Can you work these out from the model? Positions are in its coordinate system, mm. A direction names the side the tool comes from. Give positions to 0.01 mm unless a question says otherwise; leave off trailing zeros. Loops run counter-clockwise (first coordinate to the right, second up) from the corner with the lowest first, then second, coordinate; pieces in that order, holes last. Notation, with made-up numbers: (71, -8) -> (130, -8) arc R21 cw to (130, 23) -> close; hole circle Ø6 at (73, -25.75). An arc over 180 degrees is marked (long way). Use CSV: the item, a comma, the result in double quotes.
Solid Edge part; units mm, degrees
sketch "Sketch1" plane through (0, 0, 0) normal (1, 0, 0) x (0, 1, 0)
  line L0 (0, 7.4) -> (37.4, 7.4)
  line L1 (37.4, 7.4) -> (37.4, -7.4)
  line L2 (37.4, -7.4) -> (0, -7.4)
  line L3 (0, -7.4) -> (0, 7.4)
  dimension "D1" = 37.4
extrude "Protrusion1" add sketch "Sketch1" along normal mid plane 20
sketch "Sketch2" plane through (0, 0, 0) normal (0, 0, 1) x (1, 0, 0)
  line L0 (-5, 37.4) -> (-5, 46.4)
  line L1 (-5, 46.4) -> (5, 46.4)
  line L2 (5, 37.4) -> (5, 46.4)
extrude "Extrusionsausprägung_2" add sketch "Sketch2" along normal mid plane 7.8 material side at (-4.95, 41.9, 0)
fillet "Verrundung_1" radius 3 2 edges at (5, 46.4, 0) (-5, 46.4, 0)
sketch "Sketch3" plane through (0, 37.4, 0) normal (0, 1, 0) x (0, 0, -1)
  line L0 (-3.9, 5) -> (-3.9, 6.25)
  line L1 (-3.9, 6.25) -> (4.6, 6.25)
  line L2 (4.6, 6.25) -> (4.6, 5)
  line L3 (4.6, 5) -> (-3.9, 5)
  dimension "D1" = 3.9
  dimension "D2" = 3.9
extrude "Extrusionsausprägung_3" add sketch "Sketch3" along normal mid plane 2.39
sketch "Sketch4" plane through (-0.625, 41.9, 3.9) normal (0, 0, 1) x (0, 1, 0)
  circle A0 centre (-0.005, -0.625) radius 2
extrude "Cutout1" cut sketch "Sketch4" along normal mid plane 36
sketch "Sketch5" plane through (0, 18.7, 7.4) normal (0, 0, 1) x (0, 1, 0)
  line L0 (-18.7, 9.1438) -> (-10.3, 9.1438)
  line L1 (-10.3, 9.1438) -> (-8.8895, 10)
  dimension "D1" = 10.3
extrude "Extrusionsausschnitt_2" cut sketch "Sketch5" along normal mid plane 87 material side at (-9.1938, 4.2, 7.4)
sketch "Sketch6" plane through (0.4281, 0, 0) normal (0, -1, 0) x (0, 0, 1)
  circle A0 centre (0, 0.4281) radius 8
extrude "Extrusionsausprägung_4" add sketch "Sketch6" along normal blind 29.1
sketch "Sketch7" plane through (10, 18.7, 0) normal (1, 0, 0) x (0, 1, 0)
  line L0 (-55.4467, 6) -> (-18.7, 6)
  line L1 (-18.7, 6) -> (-18.7, 10.4583)
extrude "Extrusionsausschnitt_3" cut sketch "Sketch7" along normal mid plane 52 material side at (10, -18.3734, 6.05)
mirror "Mirror1" about plane through (0, 0, 0) normal (0, 0, 1) of "Extrusionsausschnitt_3"
sketch "Sketch8" plane through (0, -29.1, 0) normal (0, -1, 0) x (1, 0, 0)
  circle A0 centre (0, 0) radius 4.5
extrude "Extrusionsausschnitt_5" cut sketch "Sketch8" against normal blind 30
(1) If we section it at D-D, the plane x = 7: Write out the boundary of the cut face in (y, z).
Answer sheet:
outline,"(-29.1, -3.87) -> (0, -3.87) -> (0, -7.4) -> (37.4, -7.4) -> (37.4, 7.4) -> (0, 7.4) -> (0, 3.87) -> (-29.1, 3.87) -> close"
(2) If I drill on L1, parallel to Z at x = 0, y = -13; L2, parallel to Y at x = 0, z = 0.75 (3 decimals); L3, parallel to Y at x = 4.25, z = -5, over which ranges is the centre line in solid material (lowest first)? Write a range as from..to.
Answer sheet:
L1,"z = -6..-4.5, 4.5..6"
L2,"y = 0.9..39.895, 43.895..46.4"
L3,"y = -29.1..37.4"
(3) If we section it at C-C, the plane y = -15.5: Write out the boundary of the cut face in (x, z), then the cut area to 3 significant figures.
Answer sheet:
outline,"(-5.29, -6) -> (5.29, -6) arc R8 ccw to (5.29, 6) -> (-5.29, 6) arc R8 ccw to start; hole circle Ø9 at (0, 0)"
area,"108 mm2"
(4) Which directions (+Z, -Z, +X, -X, +Y, -Y) give clear straight access to the entire face, cutting with the end or side of a thin tool? Please do faces 1 (the face through (-1.2, 40, -3.9)), 2 (the face through (5, 40, 0)), 3 (the face through (0, -14, 6)), 4 (the face through (-6, 38.595, 0)).
Answer sheet:
face 1,"-Z, +X, +Y"
face 2,"+Z, -Z, +X, +Y"
face 3,"+Z, +X, -X, -Y"
face 4,"+Z, -Z, -X, +Y"
(5) Will these pins go through, and if not, where does the flat tip stop? pin 1 Ø10 at (x, y) = (-1.5, 41) entering from +Z; pin 2 Ø0.6 at (y, z) = (38, -2) entering from -X; pin 3 Ø6 at (y, z) = (-1, 1) entering from -X; pin 4 Ø2.5 at (x, z) = (-2, 0.5) entering from -Y.
Answer sheet:
pin 1,"stops at z = 7.4"
pin 2,"stops at x = -6.25"
pin 3,"stops at x = -9.14"
pin 4,"stops at y = 0.9"
(6) If we section it at A-A, the plane x = 0: Write out the boundary of the cut face in (y, z) (3 decimals), then the cut area to 3 significant figures.
Answer sheet:
outline,"(-29.1, -6) -> (0, -6) -> (0, -7.4) -> (37.4, -7.4) -> (37.4, -3.9) -> (39.895, -3.9) -> (39.895, 3.9) -> (37.4, 3.9) -> (37.4, 7.4) -> (0, 7.4) -> (0, 6) -> (-29.1, 6) -> (-29.1, 4.5) -> (0.9, 4.5) -> (0.9, -4.5) -> (-29.1, -4.5) -> close; (43.895, -3.9) -> (46.4, -3.9) -> (46.4, 3.9) -> (43.895, 3.9) -> close"
area,"672 mm2"
(7) We'd pull the mould along X, two halves only. Please class faces 5 (the face through (-5, 41, 0)), 6 (the face through (-0.59, -14.31, 4.46)), 7 (the face through (0, -15, -6)): released by +X, released by -X, zero draft, split by the parting line, or undercut.
Answer sheet:
face 5,"released by -X"
face 6,"undercut"
face 7,"zero draft"
